The listing builds one solid part. Answer for the finished solid, in the listing's coordinates (mm). Give positions to 0.01 mm unless a question says otherwise; leave off trailing zeros. Order: outer loops, then holes, each group sorted by start corner. A loop starts at its lowest first (then second) coordinate and runs counter-clockwise, first axis right, second up. Notation, with made-up numbers: (49, 83.25) - (65, 83.25) arc R21 cw to (65, 117.25) - close; hole circle Ø9 at (68.5, 8). An arc over 180 degrees is marked (long way). Answer as CSV lines item,"result". Start each with the question number.
1. Section D-D on x = 115 is taken. Give the vertices of the cut face in (y, z), and give its area (3 significant figures).
2. Section C-C on x = 67.5 is taken. Give the vertices of the cut face in (y, z), and give its area (3 significant figures).
3. Consider line 1 along X through (y, z) = (-47, -1.75); line 2 along Y through (x, z) = (150.5, 4.75); line 3 along X through (y, z) = (41, 3). Determine where each line is inside the solid, lowest interval first. Write a range as [from, to].
4. Section A-A on y = -10 is taken. Give the vertices of the cut face in (x, z).
5. Section B-B on x = 0 is taken. Give the vertices of the cut face in (y, z), and give its area (3 significant figures).
6. Flat-ended cylindrical pins translate along their axes: pin 1 (3 mm diameter, centred on y = 35, z = 2.5, fed in from -X); pin 2 (1.5 mm diameter, centred on y = 60, z = 3, fed in from -X); pin 3 (5 mm diameter, centred on y = 88, z = -2, fed in from -X). Find the tip coordinate at first contact, or state that the pin passes through.
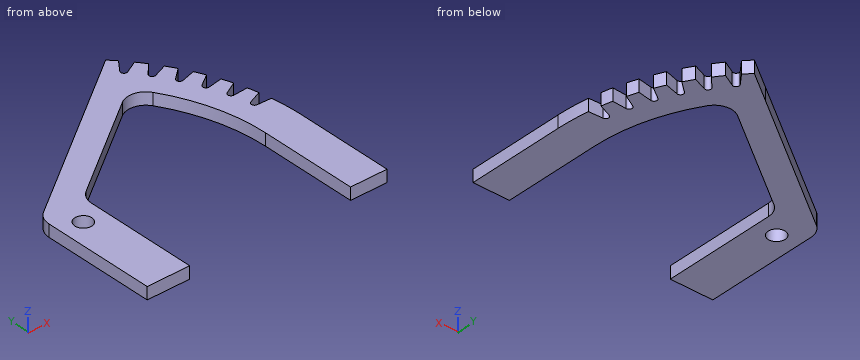
from build123d import *

# Parameters (mm, degrees)
ESQUISSE1_R        = 7
BOSS_EXTRU_2_DEPTH = 5


with BuildPart() as part:
    # Esquisse1 → Boss.-Extru.2 (new body, symmetric)
    with BuildSketch(Plane.XY):
        with BuildLine():
            Line((150, 0), (150, -80))
            Line((150, -80), (180, -80))
            Line((180, -80), (180, 0))
            ThreePointArc((180, 0), (179.515656817, 13.195793174), (178.065233806, 26.320571987))
            Line((178.065233806, 26.320571987), (166.525661597, 26.82440059))
            ThreePointArc((166.525661597, 26.82440059), (164.115561692, 28.93800148), (165.657420708, 31.748439355))
            Line((165.657420708, 31.748439355), (176.328752029, 36.168649517))
            ThreePointArc((176.328752029, 36.168649517), (175.369530112, 40.565107028), (174.300707948, 44.936212668))
            Line((174.300707948, 44.936212668), (162.772284789, 44.221349389))
            ThreePointArc((162.772284789, 44.221349389), (160.152897605, 46.069240364), (161.390047035, 49.026494422))
            Line((161.390047035, 49.026494422), (171.536232439, 54.546502735))
            ThreePointArc((171.536232439, 54.546502735), (170.119109634, 58.817416956), (168.595667923, 63.051572207))
            Line((168.595667923, 63.051572207), (157.206741362, 61.125975718))
            ThreePointArc((157.206741362, 61.125975718), (154.407228903, 62.687583949), (155.325895389, 65.758730667))
            Line((155.325895389, 65.758730667), (164.833975975, 72.317082106))
            ThreePointArc((164.833975975, 72.317082106), (162.974729307, 76.414904352), (161.013628739, 80.464969771))
            Line((161.013628739, 80.464969771), (149.89099329, 77.350078007))
            ThreePointArc((149.89099329, 77.350078007), (146.94252292, 78.608017892), (147.532478818, 81.758865764))
            Line((147.532478818, 81.758865764), (156.296599795, 89.282545285))
            ThreePointArc((156.296599795, 89.282545285), (154.015928519, 93.161653928), (151.6390023, 96.98253957))
            Line((151.6390023, 96.98253957), (140.906487819, 92.713031056))
            ThreePointArc((140.906487819, 92.713031056), (137.841885271, 93.653297773), (138.09656252, 96.84876797))
            Line((138.09656252, 96.84876797), (146.019151703, 105.254013396))
            ThreePointArc((146.019151703, 105.254013396), (143.34244685, 108.871221776), (140.576157634, 112.420389187))
            Line((140.576157634, 112.420389187), (130.353250706, 107.04379696))
            ThreePointArc((130.353250706, 107.04379696), (127.206634629, 107.655922389), (127.123197872, 110.860439292))
            Line((127.123197872, 110.860439292), (134.116051966, 120.053673851))
            ThreePointArc((134.116051966, 120.053673851), (131.415298407, 123.004143608), (128.649651075, 125.893873077))
            Line((128.649651075, 125.893873077), (104.03484123, 108.059020032))
            Line((104.03484123, 108.059020032), (-11.300992684, 24.491539248))
            ThreePointArc((-11.300992684, 24.491539248), (-15.86066784, 19.163375655), (-17.5, 12.344830732))
            Line((-17.5, 12.344830732), (-17.5, -80))
            Line((-17.5, -80), (17.5, -80))
            Line((17.5, -80), (17.5, 12.344830732))
            ThreePointArc((17.5, 12.344830732), (19.13933216, 19.163375655), (23.699007316, 24.491539248))
            Line((23.699007316, 24.491539248), (105.595221964, 83.83008228))
            ThreePointArc((105.595221964, 83.83008228), (117.258640826, 86.4077249), (127.106905164, 79.648193071))
            ThreePointArc((127.106905164, 79.648193071), (144.163164114, 41.436482871), (150, 0))
        make_face()
        Circle(ESQUISSE1_R, mode=Mode.SUBTRACT)
    extrude(amount=BOSS_EXTRU_2_DEPTH, both=True)


solid = part.part
Checks:
1,outline,"(86.67, -5) - (116, -5) - (116, 5) - (86.67, 5) - close"
1,area,"293 mm²"
2,outline,"(56.23, -5) - (81.59, -5) - (81.59, 5) - (56.23, 5) - close"
2,area,"254 mm²"
3,line 1,"x = [-17.5, 17.5], [150, 180]"
3,line 2,"y = [-80, 77.52], [84.31, 96.53]"
3,line 3,"x = [11.48, 46.48], [144.29, 175.27]"
4,outline,"(-17.5, -5) - (17.5, -5) - (17.5, 5) - (-17.5, 5) - close; (150, -5) - (180, -5) - (180, 5) - (150, 5) - close"
5,outline,"(-80, -5) - (-7, -5) - (-7, 5) - (-80, 5) - close; (7, -5) - (32.68, -5) - (32.68, 5) - (7, 5) - close"
5,area,"987 mm²"
6,pin 1,"stops at x = 1.13"
6,pin 2,"stops at x = 36.67"
6,pin 3,"stops at x = 72.9"
